The listing builds one solid part. Answer for the finished solid, in the listing's coordinates (mm). Face numbers are marked on the shaded views. A direction names the side the tool comes from. Coordinates: 2 decimals unless noted, no trailing zeros. Order: outer loops, then holes, each group sorted by start corner. A loop starts at its lowest first (then second) coordinate and runs counter-clockwise, first axis right, second up. Notation, with made-up numbers: (-9, -32) -> (21, -32) arc R16 cw to (21, -25) -> close; hole circle Ø6 at (-17, -28.5). An arc over 180 degrees is marked (long way). Write item = value, one per line.
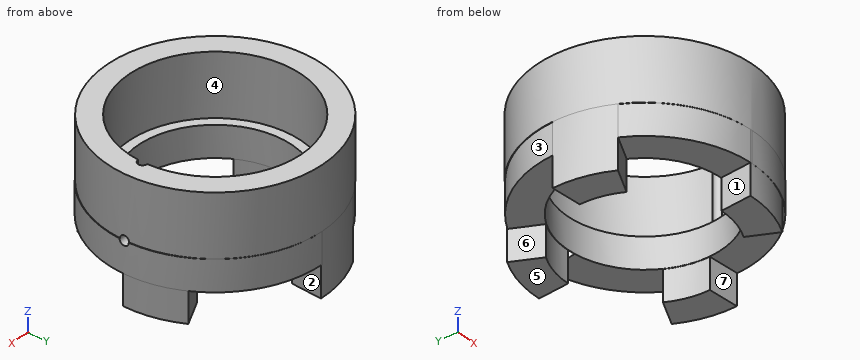
from build123d import *

# Parameters (mm, degrees)
SKETCH003_R          = 35
SKETCH003_R_2        = 28
PAD001_DEPTH         = 20
SKETCH004_R          = 35
SKETCH004_R_2        = 25
PAD002_DEPTH         = 10
PAD003_DEPTH         = 20
POLARPATTERN_COUNT   = 4
SKETCH006_R          = 1.5
POCKET002_DEPTH      = 8.5
SKETCH007_R          = 1.5
POCKET003_DEPTH      = 1
POCKET003_DEPTH_BACK = 20


with BuildPart() as part:
    # Sketch003 → Pad001 (new body)
    with BuildSketch(Plane.XY):
        Circle(SKETCH003_R)
        Circle(SKETCH003_R_2, mode=Mode.SUBTRACT)
    extrude(amount=PAD001_DEPTH)

    # Sketch004 → Pad002 (new body)
    with BuildSketch(Plane.XY):
        with Locations((0.164112, 4e-06)):
            Circle(SKETCH004_R)
        Circle(SKETCH004_R_2, mode=Mode.SUBTRACT)
    extrude(amount=-PAD002_DEPTH)

    # Sketch005 → Pad003 (new body)
    with BuildSketch(Plane.XY):
        with BuildLine():
            ThreePointArc((-34.997022, 0.456563), (-33.922695, -8.61689), (-30.536592, -17.103116))
            Line((-30.536592, -17.103116), (-21.762611, -12.504957))
            ThreePointArc((-25.093421, 0), (-24.251171, -6.471733), (-21.762611, -12.504957))
            Line((-34.997022, 0.456563), (-25.093421, 0))
        make_face()
    pad003 = extrude(amount=-PAD003_DEPTH)

    # PolarPattern: Pad003 ×4 about axis
    polarpattern_axis = Axis((0, 0, 0), (0, 0, 1))
    for i in range(1, POLARPATTERN_COUNT):
        add(pad003.rotate(polarpattern_axis, i * 360 / POLARPATTERN_COUNT))

    # Sketch006 → Pocket002 (cut, symmetric)
    with BuildSketch(Plane(origin=(35, 0, 0), x_dir=(0, 0.939693, 0.34202), z_dir=(1, 0, 0))):
        Circle(SKETCH006_R)
    extrude(amount=POCKET002_DEPTH, both=True, mode=Mode.SUBTRACT)

    # Sketch007 → Pocket003 (cut, two sides)
    with BuildSketch(Plane(origin=(28, 0, 0), x_dir=(1, 0, 0), z_dir=(0, 0, 1))) as pocket003_sk:
        Circle(SKETCH007_R)
    extrude(amount=-POCKET003_DEPTH, mode=Mode.SUBTRACT)
    extrude(pocket003_sk.sketch, amount=POCKET003_DEPTH_BACK, mode=Mode.SUBTRACT)


solid = part.part
Q1. Find the intervals of material crossed by line 1 along Y through (x, z) = (0, -5.25); line 2 along Y through (x, z) = (0, 13); line 3 along Z through (x, y) = (-26, 7), in increasing order.
The answers:
line_1 = -35 to -25, 25 to 35
line_2 = -35 to -28, 28 to 35
line_3 = -10 to 0
Q2. The mould has two halves that part along X. Classify the marked faces 5, 6 and 7: released by +X, released by -X, zero draft, split by the parting line, or undercut.
The answers:
face_5 = zero draft
face_6 = released by -X
face_7 = undercut
Q3. Each of these flat-tipped pins is pushed along its axis until it touches: pin 1 Ø10 at (x, y) = (15.5, -10) entering from +Z; pin 2 Ø10 at (x, y) = (13, 17) entering from +Z; pin 3 Ø3 at (y, z) = (4, 5.5) entering from +X; pin 4 Ø1.5 at (y, z) = (23, -6) entering from +X. Where does it stop, or does it pass through?
The answers:
pin_1 = through
pin_2 = 0
pin_3 = 34.91
pin_4 = 27.18
Q4. Section A-A, the plane z = -14.5 is taken. Give the vertices of the cut face in (x, y).
The answers:
outline = (-35, 0.46) arc R35 ccw to (-30.54, -17.1) -> (-21.76, -12.5) arc R25 cw to (-25.09, 0) -> close; (-17.1, 30.54) -> (-12.5, 21.76) arc R25 cw to (0, 25.09) -> (0.46, 35) arc R35 ccw to start; (-0.46, -35) arc R35 ccw to (17.1, -30.54) -> (12.5, -21.76) arc R25 cw to (0, -25.09) -> close; (21.76, 12.5) arc R25 cw to (25.09, 0) -> (35, -0.46) arc R35 ccw to (30.54, 17.1) -> close
Q5. Section B-B, the plane x = 19 is taken. Give the vertices of the cut face in (y, z).
The answers:
outline = (-29.5, -10) -> (-16.25, -10) -> (-16.25, 0) -> (-20.57, 0) -> (-20.57, 20) -> (-29.39, 20) -> (-29.39, 0) -> (-29.5, 0) -> close; (16.25, -10) -> (29.5, -10) -> (29.5, 0) -> (29.39, 0) -> (29.39, 20) -> (20.57, 20) -> (20.57, 0) -> (16.25, 0) -> close
Q6. A tool of negligible diameter and unlimited length cuts with its end or side. For the marked faces 1, 2, 3 and 4, from which of +Z, -Z, +X, -X, +Y, -Y can it reach the whole face along a straight path? Write none if from no direction.
The answers:
face_1 = -Z, -X
face_2 = -Z, +X
face_3 = -Z, -X, +Y
face_4 = +Z
Q7. Section C-C, the plane y = -23 is taken. Give the vertices of the cut face in (x, z), plus the area to 3 significant figures.
The answers:
outline = (-26.38, 0) -> (-26.22, 0) -> (-26.22, -10) -> (-9.8, -10) -> (-9.8, 0) -> (-15.97, 0) -> (-15.97, 20) -> (-26.38, 20) -> close; (9.8, -10) -> (10.05, -10) -> (10.05, -20) -> (13.15, -20) -> (13.15, -10) -> (26.55, -10) -> (26.55, 0) -> (26.38, 0) -> (26.38, 20) -> (15.97, 20) -> (15.97, 0) -> (9.8, 0) -> close
area = 779 mm2
